Can you work these out from the drawing? Everything is in mm from the part's minimum corner. Round coordinates to 2 decimals unless told otherwise and drop trailing zeros. Loops run counter-clockwise (first coordinate to the right, second up) from the corner with the lowest first, then second, coordinate; pieces in that order, holes last. Notation, with made-up numbers: (-11, 71) -> (36, 71) arc R30 ccw to (36, 99) -> close; hole circle Ø1 at (22.5, -28). An arc over 180 degrees is marked (long way). One line per item, written item: value.
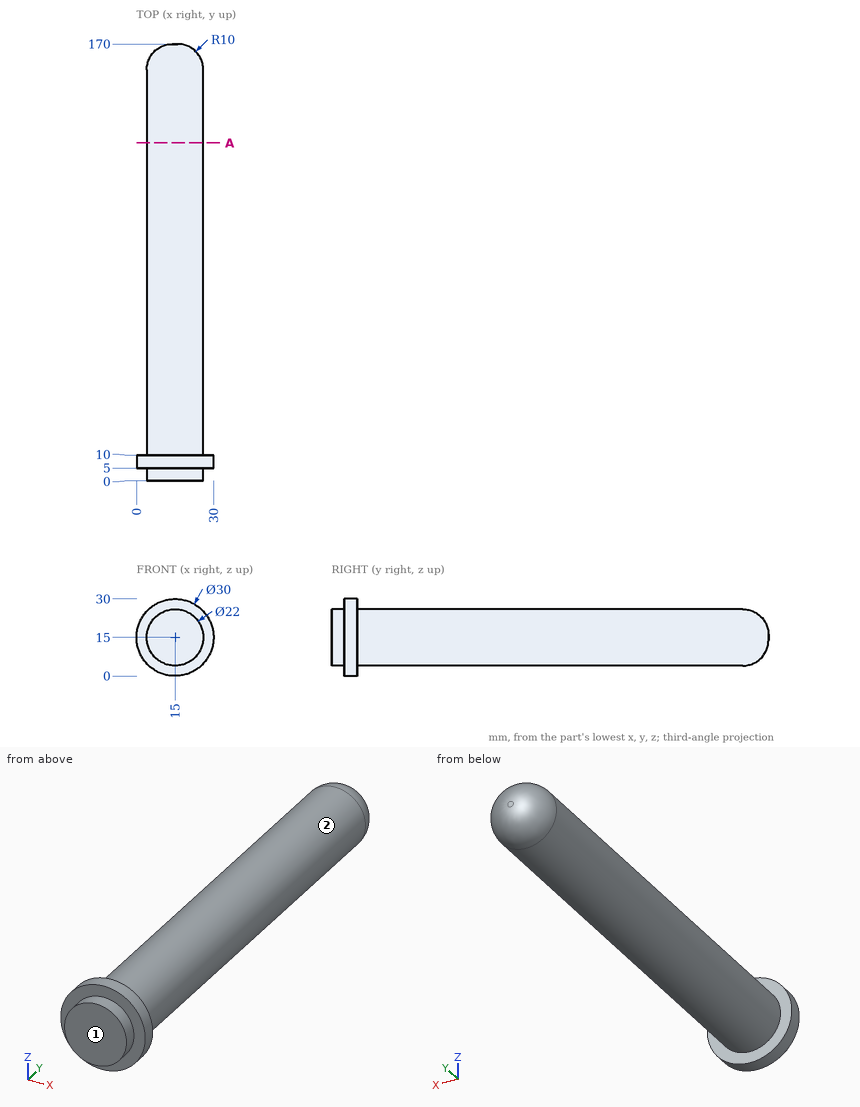
(1) Thinking about a two-plate mould opening in Y: for the marked faces 1 and 2, which applies, released by +Y, released by -Y, zero draft, split by the parting line, or undercut?
Recorded:
face 1: released by -Y
face 2: zero draft
(2) If I drill on L1, parallel to X at y = 108.5, z = 14.25; L2, parallel to Y at x = 3.25, z = 10.25; L3, parallel to X at y = 141, z = 18.5, over which ranges is the centre line in solid material (lowest first)?
Recorded:
L1: 4.03 to 25.97
L2: 5 to 10
L3: 4.57 to 25.43
(3) If we section it at A-A, the plane y = 131.5: Please give me the cut outline in (x, z), then the cut area to 3 significant figures.
Recorded:
outline: circle Ø22 at (15, 15)
area: 380 mm²
(4) I'm going to push flat-ended pins straight in: pin 1 Ø1.5 at (y, z) = (60, 14.5) entering from -X; pin 2 Ø12 at (x, y) = (14, 46.5) entering from +Z; pin 3 Ø12 at (y, z) = (61, 24) entering from -X. Where does each tip first touch, or does it pass through?
Recorded:
pin 1: x = 4
pin 2: z = 26
pin 3: x = 4.42
